Autodesk Inventor part; units mm, degrees
ref_plane "Work Plane2" through (14, -27.5, -235.8278) normal (0, 0, -1) x (0, 1, 0)
ref_plane "YZ Plane" through (0, 0, 0) normal (1, 0, 0) x (0, 1, 0)
ref_plane "XZ Plane" through (0, 0, 0) normal (0, 1, 0) x (-1, 0, 0)
ref_plane "Work Plane1" through (0, 0, 0) normal (0, 0, 1) x (1, 0, 0)
sketch "Sketch1" plane through (0, 0, 0) normal (0, 0, 1) x (1, 0, 0)
  line L0 (28.2, -13.1349) -> (28.2, -18.3349)
  arc A0 (17.8, -18.3349) -> (28.2, -18.3349) centre (23, -18.3349) ccw
  line L1 (17.8, -18.3349) -> (17.8, -13.1349)
  line L2 (17.8, -13.1349) -> (28.2, -13.1349)
  line L3 (205.8753, -18.3349) -> (205.8753, -13.1349)
  line L4 (205.8753, -13.1349) -> (216.2753, -13.1349)
  line L5 (216.2753, -13.1349) -> (216.2753, -18.3349)
  arc A1 (205.8753, -18.3349) -> (216.2753, -18.3349) centre (211.0753, -18.3349) ccw
  line L6 (226.007, -27.5) -> (182.0614, -27.5)
  line L7 (226.007, 5) -> (226.007, -27.5)
  line L8 (14, 5) -> (226.007, 5)
  line L9 (14, -27.5) -> (14, 5)
  line L10 (52.5458, -27.5) -> (14, -27.5)
  line L11 (105.8221, -25.5) -> (103.8221, -27.5)
  line L12 (105.8221, -25.5) -> (105.8221, -8.9699)
  line L13 (105.8221, -8.9699) -> (111.2221, -8.9699)
  line L14 (111.2221, -8.9699) -> (111.2221, -25.5)
  line L15 (113.2221, -27.5) -> (111.2221, -25.5)
  line L16 (151.8, -27.5) -> (113.2221, -27.5)
  line L17 (153.8, -25.5) -> (151.8, -27.5)
  line L18 (153.8, -25.5) -> (153.8, -8.9699)
  line L19 (153.8, -8.9699) -> (159.2, -8.9699)
  line L20 (159.2, -8.9699) -> (159.2, -19.6294)
  line L21 (216.0753, -18.3349) -> (216.0753, -13.3349)
  line L22 (216.0753, -13.3349) -> (206.0753, -13.3349)
  line L23 (206.0753, -13.3349) -> (206.0753, -18.3349)
  arc A2 (206.0753, -18.3349) -> (216.0753, -18.3349) centre (211.0753, -18.3349) ccw
  circle A3 centre (211.0753, -18.3349) radius 2.5
  line L24 (182.0614, -27.0054) -> (182.0614, -27.5)
  line L25 (52.5458, -27.5) -> (52.5458, -27.003)
  line L26 (52.5458, -27.003) -> (55.9407, -27.003)
  arc A4 (55.9407, -27.003) -> (66.5602, -14.9102) centre (55.9407, -16.2937) ccw
  line L27 (66.5602, -14.9102) -> (70.1135, -14.9102)
  line L28 (70.1135, -14.9102) -> (75.8231, -20.6198)
  arc A5 (72.9244, -27.5) -> (75.8231, -20.6198) centre (55.9407, -16.2937) ccw
  line L29 (103.8221, -27.5) -> (72.9244, -27.5)
  line L30 (159.2, -19.6294) -> (164.284, -14.5322)
  line L31 (164.284, -14.5322) -> (168.2242, -14.5271)
  arc A6 (168.2242, -14.5271) -> (178.6664, -27.0054) centre (178.6664, -16.397) ccw
  line L32 (178.6664, -27.0054) -> (182.0614, -27.0054)
  circle A7 centre (55.9407, -16.2937) radius 1.5
  circle A8 centre (178.6664, -16.397) radius 1.5
  point P0 (0, 0)
  dimension "d0" = 0.2
  dimension "d1" = 5
ref_plane "Work Plane2" through (14, -27.5, -235.8278) normal (0, 0, -1) x (0, 1, 0)
extrude "Extrusion1" add sketch "Sketch1" against normal up to surface (235.8278 mm away) contours A2 L23 L22 L21
properties part number "BaseShaft_3DPrint"
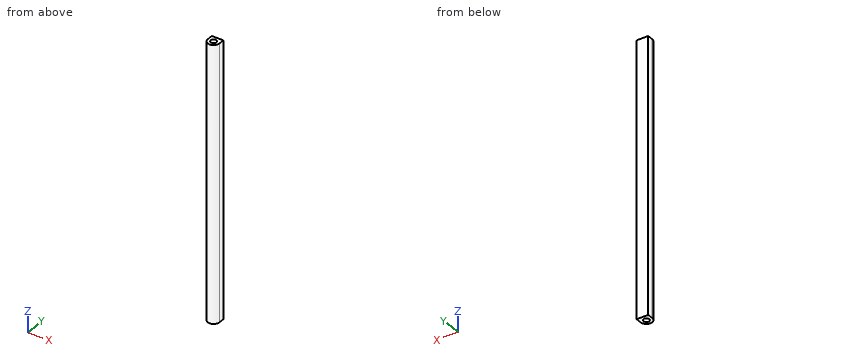
Could you check a few things on this model? Use its own coordinates, in mm. Give positions to 0.01 mm unless a question says otherwise; leave off trailing zeros. Order: outer loops, then holes, each group sorted by start corner. A loop starts at its lowest first (then second) coordinate and runs counter-clockwise, first axis right, second up. Notation, with made-up numbers: (1.25, 36.5) -> (55.25, 36.5) arc R26 cw to (55.25, 61.5) -> close; hole circle Ø7 at (35, 63). An arc over 180 degrees is marked (long way). Return JSON: item names as keys, results as strings.
1. For pin 1 Ø5 at (x, z) = (214, -78) entering from -Y; pin 2 Ø3 at (x, z) = (214, -51.5) entering from -Y; pin 3 Ø5 at (x, y) = (214, -17) entering from +Z, each with a flat end and sliding along its axis, tell me the tip position at first contact or that it passes through.
Answer list:
{"pin 1": "stops at y = -23.32", "pin 2": "stops at y = -23.13", "pin 3": "stops at z = 0"}
2. I need wall thicknesses on line 1 (Y direction, x = 211.5, z = -50); line 2 (X direction, y = -18.75, z = -164); line 3 (X direction, y = -18.25, z = -184.5). Which ranges of each line are inside material? Lowest first, please. Write a range as from..to.
Answer list:
{"line 1": "y = -23.32..-20.8, -15.87..-13.33", "line 2": "x = 206.09..208.61, 213.54..216.06", "line 3": "x = 206.08..208.58, 213.57..216.08"}
3. Imagine slicing it at A-A on z = -52.5. List the corners of the cut face in (x, y) for me.
Answer list:
{"outline": "(206.08, -18.33) arc R5 ccw to (216.08, -18.33) -> (216.08, -13.33) -> (206.08, -13.33) -> close; hole circle Ø5 at (211.08, -18.33)"}
